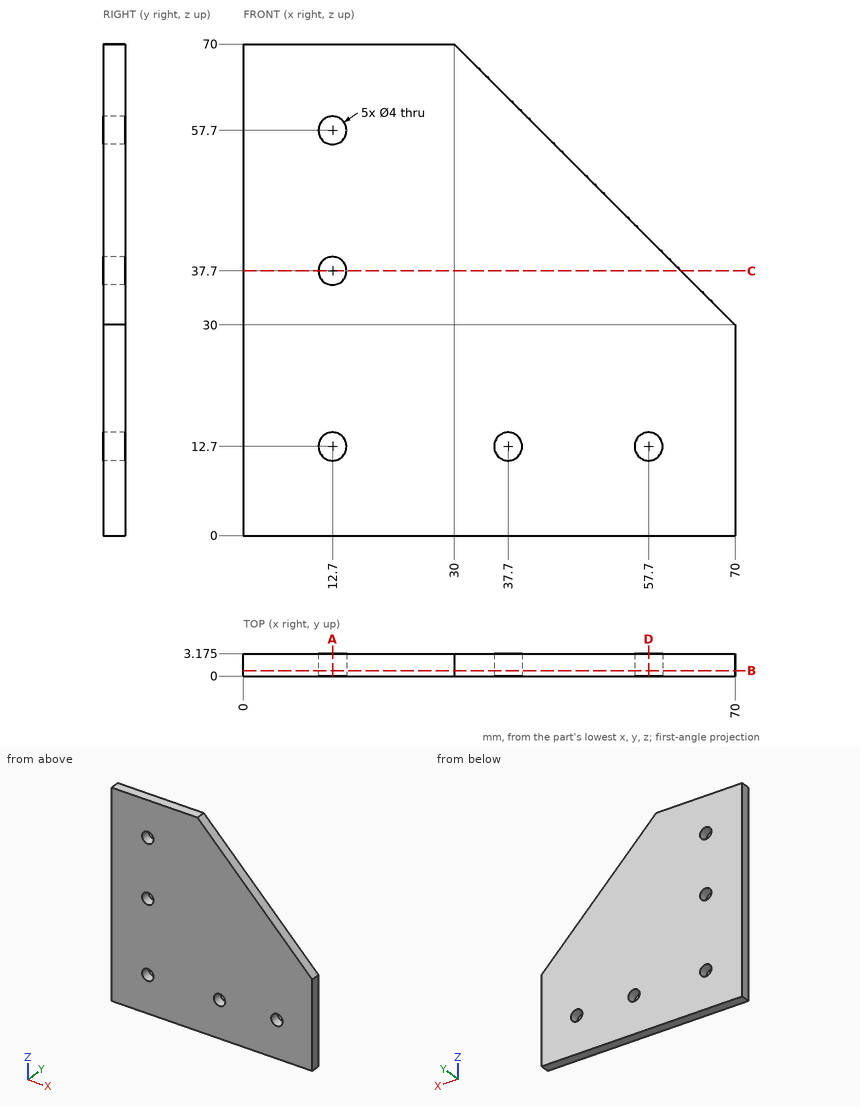
Job drawing, mm, ordinate dimensions from the low corner. One solid piece. Coordinates: 2 decimals unless noted, no trailing zeros. Write each loop counter-clockwise with the first axis right and the second up, starting at its lowest first coordinate (ties: lowest second). Pieces come first, ordered by that corner, then holes.
Item 1: Slice it at B-B (y = 0.75). Write the cut outline in (x, z).
Item 2: Slice it at A-A (x = 12.7). Write the cut outline in (y, z) (3 decimals), and give its area (3 significant figures).
Item 3: Pin check, flat tip, straight feed: pin 1 (3 mm diameter, centred on x = 37.7, z = 12.7, fed in from -Y). Stop position of the tip, or through.
Item 4: Probe line 1 (X direction, y = 0.85, z = 12.7); line 2 (X direction, y = 1.4, z = 56). List the from-to ranges inside material, lowest first.
Item 5: Slice it at D-D (x = 57.7). Write the cut outline in (y, z) (3 decimals), and give its area (3 significant figures).
Item 6: Slice it at C-C (z = 37.7). Write the cut outline in (x, y) (3 decimals), and give its area (3 significant figures).
Results found:
1. outline: (0, 0) - (70, 0) - (70, 30) - (30, 70) - (0, 70) - close; hole circle Ø4 at (12.7, 12.7); hole circle Ø4 at (12.7, 37.7); hole circle Ø4 at (12.7, 57.7); hole circle Ø4 at (37.7, 12.7); hole circle Ø4 at (57.7, 12.7)
2. outline: (0, 0) - (3.175, 0) - (3.175, 10.7) - (0, 10.7) - close; (0, 14.7) - (3.175, 14.7) - (3.175, 35.7) - (0, 35.7) - close; (0, 39.7) - (3.175, 39.7) - (3.175, 55.7) - (0, 55.7) - close; (0, 59.7) - (3.175, 59.7) - (3.175, 70) - (0, 70) - close
2. area: 184 mm2
3. pin 1: passes through
4. line 1: x = 0 to 10.7, 14.7 to 35.7, 39.7 to 55.7, 59.7 to 70
4. line 2: x = 0 to 11.65, 13.75 to 44
5. outline: (0, 0) - (3.175, 0) - (3.175, 10.7) - (0, 10.7) - close; (0, 14.7) - (3.175, 14.7) - (3.175, 42.3) - (0, 42.3) - close
5. area: 122 mm2
6. outline: (0, 0) - (10.7, 0) - (10.7, 3.175) - (0, 3.175) - close; (14.7, 0) - (62.3, 0) - (62.3, 3.175) - (14.7, 3.175) - close
6. area: 185 mm2
